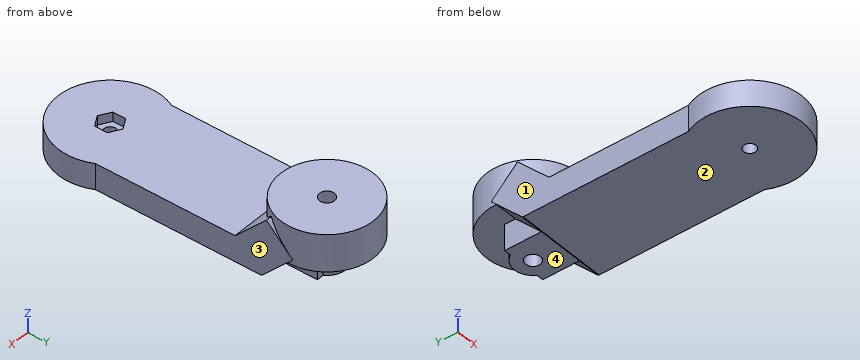
```python
from build123d import *

# Parameters (mm, degrees)
F1_DEPTH  = 7
F2_R      = 12.5
F3_DEPTH  = 10
F4_R      = 2
F5_DEPTH  = 7
F9_W      = 25
F9_H      = 12
F10_DEPTH = 10
F11_R     = 2
F12_DEPTH = 17
F13_R     = 14
F14_DEPTH = 7
F15_R     = 1.65
F16_DEPTH = 7
F18_DEPTH = 2.5


with BuildPart() as f1:
    # F0 (on Top) → F1 (new body)
    with BuildSketch(Plane.XY):
        Polygon((-12.5, -27.5), (12.5, -27.5), (12.5, 27.5), (6.25, 27.5), (-6.25, 27.5), (-12.5, 27.5), align=None)
        with BuildLine():
            Line((-6.25, 27.5), (6.25, 27.5))
            Line((6.25, 27.5), (6.25, 37.5))
            Line((6.25, 37.5), (4.3301270189, 37.5))
            ThreePointArc((4.3301270189, 37.5), (4.8296291314, 36.2940952255), (5, 35))
            ThreePointArc((5, 35), (-1.2940952255, 30.1703708686), (-4.3301270189, 37.5))
            Line((-4.3301270189, 37.5), (-6.25, 37.5))
            Line((-6.25, 37.5), (-6.25, 27.5))
        make_face()
        with BuildLine():
            ThreePointArc((5, 35), (4.8296291314, 36.2940952255), (4.3301270189, 37.5))
            Line((4.3301270189, 37.5), (-4.3301270189, 37.5))
            ThreePointArc((-4.3301270189, 37.5), (-1.2940952255, 30.1703708686), (5, 35))
        make_face()
        with BuildLine():
            Line((-4.3301270189, 37.5), (4.3301270189, 37.5))
            ThreePointArc((4.3301270189, 37.5), (0, 40), (-4.3301270189, 37.5))
        make_face()
    extrude(amount=F1_DEPTH)

    # F2 (on face) → F3 (join)
    with BuildSketch(Plane.XY.offset(7)):
        with Locations((0, 35)):
            Circle(F2_R)
    extrude(amount=F3_DEPTH)

    # F4 (on face) → F5 (cut, through all)
    with BuildSketch(Plane.XY.offset(7)):
        with Locations((0, -23.5)):
            Circle(F4_R)
    extrude(amount=-F5_DEPTH, mode=Mode.SUBTRACT)

    # F9 (on offset) → F10 (join)
    with BuildSketch(Plane(origin=(0, 6.7144660941, -6.7144660941), x_dir=(1, 0, 0), z_dir=(0, -0.7071067812, 0.7071067812))):
        with Locations((0, 25.3951839509)):
            Rectangle(F9_W, F9_H)
    extrude(amount=-F10_DEPTH)

    # F11 (on face) → F12 (cut, through all)
    with BuildSketch(Plane.XY.offset(17)):
        with Locations((0, 35)):
            Circle(F11_R)
    extrude(amount=-F12_DEPTH, mode=Mode.SUBTRACT)

    # F13 (on face) → F14 (join, through all)
    with BuildSketch(Plane(origin=(0, 0, 0), x_dir=(1, 0, 0), z_dir=(0, 0, -1))):
        with Locations((0, 23.5)):
            Circle(F13_R)
    extrude(amount=-F14_DEPTH)

    # F15 (on face) → F16 (cut, through all)
    with BuildSketch(Plane.XY.offset(7)):
        with Locations((0, -23.5)):
            Circle(F15_R)
    extrude(amount=-F16_DEPTH, mode=Mode.SUBTRACT)

    # F17 (on face) → F18 (cut)
    with BuildSketch(Plane.XY.offset(7)):
        Polygon((0, -26.9641016151), (3, -25.2320508076), (3, -21.7679491924), (0, -20.0358983849), (-3, -21.7679491924), (-3, -25.2320508076), align=None)
    extrude(amount=-F18_DEPTH, mode=Mode.SUBTRACT)


solid = f1.part
```
Geometry check sheet. Reference: the model listing, model coordinates, mm. Face numbers are marked on the shaded views. A direction names the side the tool comes from. Coordinates: 2 decimals unless noted, no trailing zeros. Loops run counter-clockwise (first coordinate to the right, second up) from the corner with the lowest first, then second, coordinate; pieces in that order, holes last.
Item 1: Sectioned sample at A-A, the plane y = -23.5. Record the boundary of the cut face in (x, z), then the cut area to 3 significant figures.
Item 2: Access from +Z, -Z, +X, -X, +Y, -Y to the whole of each face (thin tool, end or side, straight path). Record for the marked faces 1, 2, 3 and 4.
Item 3: Sectioned sample at D-D, the plane x = 7.25. Record the boundary of the cut face in (y, z), then the cut area to 3 significant figures.
Item 4: Sectioned sample at B-B, the plane z = 14.75. Record the boundary of the cut face in (x, y).
Item 5: Sectioned sample at C-C, the plane z = 6.25. Record the boundary of the cut face in (x, y), then the cut area to 3 significant figures.
Item 6: Thickness scan on line 1 (Y direction, x = 0, z = 11.5); line 2 (Z direction, x = 4, y = 37); line 3 (Z direction, x = -7, y = -27). Record the ranges inside material, lowest first.
Item 7: Go/stop test with flat-tipped pins: pin 1 Ø3 at (x, z) = (8.5, 6.5) entering from +Y; pin 2 Ø2 at (x, y) = (6, 2.5) entering from +Z; pin 3 Ø5 at (x, y) = (0, 35) entering from +Z; pin 4 Ø8.5 at (x, y) = (-6, -4.5) entering from -Z. Record where each tip stops, or that it passes through.
Check result:
1. outline: (-14, 0) - (-1.65, 0) - (-1.65, 4.5) - (-3, 4.5) - (-3, 7) - (-14, 7) - close; (1.65, 0) - (14, 0) - (14, 7) - (3, 7) - (3, 4.5) - (1.65, 4.5) - close
1. area: 166 mm2
2. face 1: +Z, -Z, -X, +Y
2. face 2: -Z, +X, -X, -Y
2. face 3: +Z, -Z, +X, +Y
2. face 4: -Z, +X, -X, +Y
3. outline: (-35.48, 0) - (27.43, 0) - (27.5, -0.07) - (34.57, 7) - (45.18, 7) - (45.18, 17) - (24.82, 17) - (24.82, 11.39) - (20.43, 7) - (-35.48, 7) - close
3. area: 679 mm2
4. outline: (-12.5, 28.18) - (-10.47, 28.18) arc R12.5 ccw to (10.47, 28.18) - (12.5, 28.18) - (12.5, 29.65) - (11.3, 29.65) arc R12.5 ccw (long way) to (-11.3, 29.65) - (-12.5, 29.65) - close; hole circle Ø4 at (0, 35)
5. outline: (-12.5, -17.2) arc R14 ccw (long way) to (12.5, -17.2) - (12.5, 33.82) - (6.25, 33.82) - (6.25, 37.5) - (4.33, 37.5) arc R5 ccw to (-4.33, 37.5) - (-6.25, 37.5) - (-6.25, 33.82) - (-12.5, 33.82) - close; hole (-3, -25.23) - (0, -26.96) - (3, -25.23) - (3, -21.77) - (0, -20.04) - (-3, -21.77) - close; hole circle Ø4 at (0, 35)
5. area: 1,770 mm2
6. line 1: y = 22.5 to 33, 37 to 47.5
6. line 2: z = 0 to 17
6. line 3: z = 0 to 7
7. pin 1: stops at y = 45.3
7. pin 2: stops at z = 7
7. pin 3: stops at z = 17
7. pin 4: stops at z = 0
